```python
from build123d import *

# Parameters (mm, degrees)
BOSS_EXTRUDE1_DEPTH = 23
CUT_EXTRUDE1_DEPTH  = 76
CHAMFER1_SIZE       = 2
CUT_EXTRUDE2_START  = -68
SKETCH4_R           = 6
SKETCH4_W           = 28
SKETCH4_H           = 28
SKETCH4_W_2         = 3
CUT_EXTRUDE2_DEPTH  = 2
SKETCH4_3_R         = 6
CUT_EXTRUDE3_DEPTH  = 127.368508735
CUT_EXTRUDE4_START  = -66
SKETCH4_4_R         = 6
SKETCH4_4_W         = 28
SKETCH4_4_H         = 28
CUT_EXTRUDE4_DEPTH  = 10
CHAMFER2_SIZE       = 1
FILLET1_R           = 8


with BuildPart() as part:
    # Sketch1 → Boss-Extrude1 (new, symmetric)
    with BuildSketch(Plane.XY):
        with BuildLine():
            Line((-104, 0), (104, 0))
            Line((104, 0), (99.985564599, 14))
            Line((99.985564599, 14), (54, 14))
            Line((54, 14), (54, 68))
            Line((54, 68), (28, 68))
            Line((28, 68), (28, 52))
            Line((28, 52), (24, 52))
            Line((24, 52), (24, 48))
            ThreePointArc((24, 48), (0, 24), (-24, 48))
            Line((-24, 48), (-24, 52))
            Line((-24, 52), (-28, 52))
            Line((-28, 52), (-28, 68))
            Line((-28, 68), (-54, 68))
            Line((-54, 68), (-54, 14))
            Line((-54, 14), (-99.985564599, 14))
            Line((-99.985564599, 14), (-104, 0))
        make_face()
    extrude(amount=BOSS_EXTRUDE1_DEPTH, both=True)

    # Sketch3 → Cut-Extrude1 (cut)
    with BuildSketch(Plane(origin=(0, 14, 0), x_dir=(1, 0, 0), z_dir=(0, 1, 0))):
        with BuildLine():
            Line((-48.856934001, 23), (-54, 23))
            Line((-54, 23), (-54, 2.63e-07))
            ThreePointArc((-54, 2.63e-07), (-52.698550407, 11.784005473), (-48.856934001, 23))
        make_face()
        with BuildLine():
            ThreePointArc((-48.856934001, -23), (-52.698550464, -11.784005217), (-54, 2.63e-07))
            Line((-54, 2.63e-07), (-54, -23))
            Line((-54, -23), (-48.856934001, -23))
        make_face()
        with BuildLine():
            Line((48.856934001, -23), (54, -23))
            Line((54, -23), (54, 0))
            ThreePointArc((54, 0), (52.698550436, -11.784005345), (48.856934001, -23))
        make_face()
        with BuildLine():
            ThreePointArc((48.856934001, 23), (52.698550436, 11.784005345), (54, 0))
            Line((54, 0), (54, 23))
            Line((54, 23), (48.856934001, 23))
        make_face()
    extrude(amount=CUT_EXTRUDE1_DEPTH, mode=Mode.SUBTRACT)

    # Chamfer1
    chamfer1_edges = [part.edges().sort_by_distance(p)[0] for p in [
        (-24, 50, -23),
        (0, 24, -23),
        (24, 50, -23),
        (24, 50, 23),
        (0, 24, 23),
        (-24, 50, 23),
    ]]
    chamfer(chamfer1_edges, length=CHAMFER1_SIZE)

    # Sketch4 → Cut-Extrude2 (cut)
    # profile 1 of 14: a face of its own
    with BuildSketch(Plane(origin=(0, 68, 0), x_dir=(1, 0, 0), z_dir=(0, 1, 0)).offset(CUT_EXTRUDE2_START)):
        with BuildLine():
            Line((-53, 10.344080433), (-53, 14))
            Line((-53, 14), (-52.153619242, 14))
            ThreePointArc((-52.153619242, 14), (-51.649321328, 15.759048395), (-51.085712288, 17.5))
            Line((-51.085712288, 17.5), (-97.5, 17.5))
            Line((-97.5, 17.5), (-97.5, -17.5))
            Line((-97.5, -17.5), (-51.085712288, -17.5))
            ThreePointArc((-51.085712288, -17.5), (-51.649321328, -15.759048395), (-52.153619242, -14))
            Line((-52.153619242, -14), (-53, -14))
            Line((-53, -14), (-53, -10.344080433))
            ThreePointArc((-53, -10.344080433), (-54, 0), (-53, 10.344080433))
        make_face()
        with BuildLine():
            ThreePointArc((-85, -6), (-91, 0), (-85, 6))
            Line((-85, 6), (-77, 6))
            ThreePointArc((-77, 6), (-71, 0), (-77, -6))
            Line((-77, -6), (-85, -6))
        make_face(mode=Mode.SUBTRACT)
    # profile 2 of 14: a face of its own
    with BuildSketch(Plane(origin=(0, 68, 0), x_dir=(1, 0, 0), z_dir=(0, 1, 0)).offset(CUT_EXTRUDE2_START)):
        with BuildLine():
            Line((-28, 14), (-52.153619242, 14))
            ThreePointArc((-52.153619242, 14), (-52.608576743, 12.179394612), (-53, 10.344080433))
            Line((-53, 10.344080433), (-53, -10.344080433))
            ThreePointArc((-53, -10.344080433), (-52.608576743, -12.179394612), (-52.153619242, -14))
            Line((-52.153619242, -14), (-28, -14))
            Line((-28, -14), (-28, 14))
        make_face()
        with Locations((-39, 0)):
            Circle(SKETCH4_R, mode=Mode.SUBTRACT)
    # profile 3 of 14: a face of its own
    with BuildSketch(Plane(origin=(0, 68, 0), x_dir=(1, 0, 0), z_dir=(0, 1, 0)).offset(CUT_EXTRUDE2_START)):
        with Locations((-39, 0)):
            Circle(SKETCH4_R)
    # profile 4 of 14: a face of its own
    with BuildSketch(Plane(origin=(0, 68, 0), x_dir=(1, 0, 0), z_dir=(0, 1, 0)).offset(CUT_EXTRUDE2_START)):
        with BuildLine():
            Line((-85, -6), (-77, -6))
            ThreePointArc((-77, -6), (-71, 0), (-77, 6))
            Line((-77, 6), (-85, 6))
            ThreePointArc((-85, 6), (-91, 0), (-85, -6))
        make_face()
    # profile 5 of 14: a face of its own
    with BuildSketch(Plane(origin=(0, 68, 0), x_dir=(1, 0, 0), z_dir=(0, 1, 0)).offset(CUT_EXTRUDE2_START)):
        with BuildLine():
            Line((-28, -17.5), (-28, -14))
            Line((-28, -14), (-52.153619242, -14))
            ThreePointArc((-52.153619242, -14), (-51.649321328, -15.759048395), (-51.085712288, -17.5))
            Line((-51.085712288, -17.5), (-28, -17.5))
        make_face()
    # profile 6 of 14: a face of its own
    with BuildSketch(Plane(origin=(0, 68, 0), x_dir=(1, 0, 0), z_dir=(0, 1, 0)).offset(CUT_EXTRUDE2_START)):
        with BuildLine():
            ThreePointArc((-51.085712288, 17.5), (-51.649321328, 15.759048395), (-52.153619242, 14))
            Line((-52.153619242, 14), (-28, 14))
            Line((-28, 14), (-28, 17.5))
            Line((-28, 17.5), (-51.085712288, 17.5))
        make_face()
    # profile 7 of 14: a face of its own
    with BuildSketch(Plane(origin=(0, 68, 0), x_dir=(1, 0, 0), z_dir=(0, 1, 0)).offset(CUT_EXTRUDE2_START)):
        Polygon((-28, 17.5), (-28, 14), (-25, 14), (-25, -14), (-28, -14), (-28, -17.5), (97.5, -17.5), (97.5, 17.5), align=None)
        with Locations((39, 0)):
            Rectangle(SKETCH4_W, SKETCH4_H, mode=Mode.SUBTRACT)
        with BuildLine():
            Line((77, 6), (85, 6))
            ThreePointArc((85, 6), (91, 0), (85, -6))
            Line((85, -6), (77, -6))
            ThreePointArc((77, -6), (71, 0), (77, 6))
        make_face(mode=Mode.SUBTRACT)
    # profile 8 of 14: a face of its own
    with BuildSketch(Plane(origin=(0, 68, 0), x_dir=(1, 0, 0), z_dir=(0, 1, 0)).offset(CUT_EXTRUDE2_START)):
        with BuildLine():
            ThreePointArc((-52.153619242, -14), (-52.608576743, -12.179394612), (-53, -10.344080433))
            Line((-53, -10.344080433), (-53, -14))
            Line((-53, -14), (-52.153619242, -14))
        make_face()
    # profile 9 of 14: a face of its own
    with BuildSketch(Plane(origin=(0, 68, 0), x_dir=(1, 0, 0), z_dir=(0, 1, 0)).offset(CUT_EXTRUDE2_START)):
        with BuildLine():
            Line((-53, -10.344080433), (-53, 10.344080433))
            ThreePointArc((-53, 10.344080433), (-54, 0), (-53, -10.344080433))
        make_face()
    # profile 10 of 14: a face of its own
    with BuildSketch(Plane(origin=(0, 68, 0), x_dir=(1, 0, 0), z_dir=(0, 1, 0)).offset(CUT_EXTRUDE2_START)):
        with BuildLine():
            Line((-52.153619242, 14), (-53, 14))
            Line((-53, 14), (-53, 10.344080433))
            ThreePointArc((-53, 10.344080433), (-52.608576743, 12.179394612), (-52.153619242, 14))
        make_face()
    # profile 11 of 14: a face of its own
    with BuildSketch(Plane(origin=(0, 68, 0), x_dir=(1, 0, 0), z_dir=(0, 1, 0)).offset(CUT_EXTRUDE2_START)):
        with Locations((-26.5, 0)):
            Rectangle(SKETCH4_W_2, SKETCH4_H)
    # profile 12 of 14: a face of its own
    with BuildSketch(Plane(origin=(0, 68, 0), x_dir=(1, 0, 0), z_dir=(0, 1, 0)).offset(CUT_EXTRUDE2_START)):
        with BuildLine():
            ThreePointArc((77, -6), (71, 0), (77, 6))
            Line((77, 6), (85, 6))
            ThreePointArc((85, 6), (91, 0), (85, -6))
            Line((85, -6), (77, -6))
        make_face()
    # profile 13 of 14: a face of its own
    with BuildSketch(Plane(origin=(0, 68, 0), x_dir=(1, 0, 0), z_dir=(0, 1, 0)).offset(CUT_EXTRUDE2_START)):
        with Locations((39, 0)):
            Rectangle(SKETCH4_W, SKETCH4_H)
        with Locations((39, 0)):
            Circle(SKETCH4_R, mode=Mode.SUBTRACT)
    # profile 14 of 14: a face of its own
    with BuildSketch(Plane(origin=(0, 68, 0), x_dir=(1, 0, 0), z_dir=(0, 1, 0)).offset(CUT_EXTRUDE2_START)):
        with Locations((39, 0)):
            Circle(SKETCH4_R)
    extrude(amount=CUT_EXTRUDE2_DEPTH, mode=Mode.SUBTRACT)

    # Sketch4<3> → Cut-Extrude3 (cut, through all)
    with BuildSketch(Plane(origin=(0, 68, 0), x_dir=(1, 0, 0), z_dir=(0, 1, 0))):
        with Locations(Location((-39, 0, 0), (0, 0, 270))):
            Circle(SKETCH4_3_R)
        with Locations(Location((39, 0, 0), (0, 0, 270))):
            Circle(SKETCH4_3_R)
        with BuildLine():
            Line((-85, -6), (-77, -6))
            ThreePointArc((-77, -6), (-71, 0), (-77, 6))
            Line((-77, 6), (-85, 6))
            ThreePointArc((-85, 6), (-91, 0), (-85, -6))
        make_face()
        with BuildLine():
            ThreePointArc((77, -6), (71, 0), (77, 6))
            Line((77, 6), (85, 6))
            ThreePointArc((85, 6), (91, 0), (85, -6))
            Line((85, -6), (77, -6))
        make_face()
    extrude(amount=-CUT_EXTRUDE3_DEPTH, mode=Mode.SUBTRACT)

    # Sketch4<4> → Cut-Extrude4 (cut)
    # profile 1 of 4: a face of its own
    with BuildSketch(Plane(origin=(0, 68, 0), x_dir=(1, 0, 0), z_dir=(0, 1, 0)).offset(CUT_EXTRUDE4_START)):
        with BuildLine():
            Line((-28, 14), (-52.153619242, 14))
            ThreePointArc((-52.153619242, 14), (-52.608576743, 12.179394612), (-53, 10.344080433))
            Line((-53, 10.344080433), (-53, -10.344080433))
            ThreePointArc((-53, -10.344080433), (-52.608576743, -12.179394612), (-52.153619242, -14))
            Line((-52.153619242, -14), (-28, -14))
            Line((-28, -14), (-28, 14))
        make_face()
        with Locations(Location((-39, 0, 0), (0, 0, 270))):
            Circle(SKETCH4_4_R, mode=Mode.SUBTRACT)
    # profile 2 of 4: a face of its own
    with BuildSketch(Plane(origin=(0, 68, 0), x_dir=(1, 0, 0), z_dir=(0, 1, 0)).offset(CUT_EXTRUDE4_START)):
        with Locations((39, 0)):
            Rectangle(SKETCH4_4_W, SKETCH4_4_H)
        with Locations(Location((39, 0, 0), (0, 0, 270))):
            Circle(SKETCH4_4_R, mode=Mode.SUBTRACT)
    # profile 3 of 4: a face of its own
    with BuildSketch(Plane(origin=(0, 68, 0), x_dir=(1, 0, 0), z_dir=(0, 1, 0)).offset(CUT_EXTRUDE4_START)):
        with Locations(Location((-39, 0, 0), (0, 0, 270))):
            Circle(SKETCH4_4_R)
    # profile 4 of 4: a face of its own
    with BuildSketch(Plane(origin=(0, 68, 0), x_dir=(1, 0, 0), z_dir=(0, 1, 0)).offset(CUT_EXTRUDE4_START)):
        with Locations(Location((39, 0, 0), (0, 0, 270))):
            Circle(SKETCH4_4_R)
    extrude(amount=CUT_EXTRUDE4_DEPTH, mode=Mode.SUBTRACT)

    # Chamfer2
    chamfer2_edges = [part.edges().sort_by_distance(p)[0] for p in [
        (71, 14, 0),
        (81, 14, -6),
        (91, 14, 0),
        (81, 14, 6),
        (-81, 14, 6),
        (-91, 14, 0),
        (-81, 14, -6),
        (-71, 14, 0),
    ]]
    chamfer(chamfer2_edges, length=CHAMFER2_SIZE)

    # Fillet1
    fillet1_edges = [part.edges().sort_by_distance(p)[0] for p in [
        (-54, 14, 0),
        (54, 14, 0),
    ]]
    fillet(fillet1_edges, radius=FILLET1_R)


solid = part.part
```
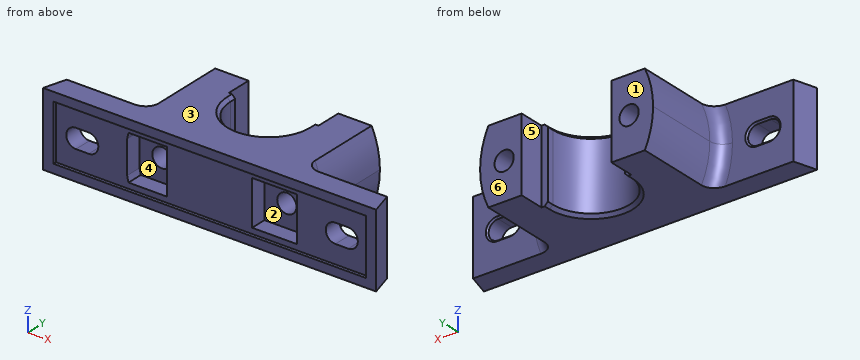
Can you work these out from the model? Positions are in its coordinate system, mm. Face numbers are marked on the shaded views. A direction names the side the tool comes from. Coordinates: 2 decimals unless noted, no trailing zeros. Order: outer loops, then holes, each group sorted by start corner. A loop starts at its lowest first (then second) coordinate and runs counter-clockwise, first axis right, second up.
1. I need wall thicknesses on line 1 (X direction, y = 55.5, z = 0); line 2 (X direction, y = 28.5, z = 0); line 3 (X direction, y = 3.5, z = 10.5). Which ranges of each line are inside material? Lowest first, please.
2. If we section it at A-A (y = 56): Please give me the cut outline in (x, z), then the cut area to 3 significant figures.
3. I'm going to push flat-ended pins straight in: pin 1 (5 mm diameter, centred on y = 6, z = 1.5, fed in from -X); pin 2 (13 mm diameter, centred on y = 56, z = -4, fed in from +X); pin 3 (4.5 mm diameter, centred on x = 26, z = 3.5, fed in from +Y); pin 4 (4.5 mm diameter, centred on y = 49.5, z = 5.5, fed in from +X). Where does each tip first touch, or does it pass through?
4. If we section it at B-B (x = -39): Please give me the cut outline in (y, z), then the cut area to 3 significant figures.
5. For the marked faces 4, 5 and 6, which set-ups out of +Z, -Z, +X, -X, +Y, -Y let a thin tool reach every point of the face, with its end or its side?
6. If we section it at D-D (y = 20): Please give me the cut outline in (x, z).
7. If we section it at C-C (x = 0): Please give me the cut outline in (y, z).
8. Thinking about a two-plate mould opening in Z: for the marked faces 1, 2 and 3, which applies, +Z half, -Z half, draft (parallel to the pull), parting line (faces both ways), or undercut?
Entries:
1. line 1: x = -54 to -45, -33 to -28, 28 to 33, 45 to 54
1. line 2: x = -54 to -45, -33 to -13.99, 13.99 to 33, 45 to 54
1. line 3: x = -103 to -52.97, -28 to 25, 53 to 103
2. outline: (-48.86, -23) - (-28, -23) - (-28, 23) - (-48.86, 23) arc R54 ccw to start; (28, -23) - (48.86, -23) arc R54 ccw to (48.86, 23) - (28, 23) - close; hole circle Ø12 at (-39, 0); hole circle Ø12 at (39, 0)
2. area: 2,010 mm2
3. pin 1: stops at x = -103
3. pin 2: stops at x = 54
3. pin 3: stops at y = 68
3. pin 4: stops at x = 53.9
4. outline: (0, -23) - (68, -23) - (68, -6) - (12, -6) - (12, -14) - (2, -14) - (2, -17.5) - (0, -17.5) - close; (0, 17.5) - (2, 17.5) - (2, 14) - (12, 14) - (12, 6) - (68, 6) - (68, 23) - (0, 23) - close
4. area: 2,110 mm2
5. face 4: -Y
5. face 5: +Z, -Z, +Y
5. face 6: +Z, -Z, +X, -X, +Y
6. outline: (-49.14, -23) - (49.14, -23) arc R54.25 ccw to (49.14, 23) - (-49.14, 23) arc R54.25 ccw to start; hole circle Ø12 at (-39, 0); hole circle Ø12 at (39, 0)
7. outline: (0, -23) - (22, -23) - (24, -21) - (24, 21) - (22, 23) - (0, 23) - (0, 17.5) - (2, 17.5) - (2, -17.5) - (0, -17.5) - close
8. face 1: draft
8. face 2: undercut
8. face 3: +Z half
